For this review, take the finished solid that the model builds, in its own axes (mm). Face numbers are marked on the shaded views. A direction names the side the tool comes from. Give positions to 0.01 mm unless a question says otherwise; leave off trailing zeros. Write each loop counter-clockwise with the first axis right and the second up, starting at its lowest first coordinate (ties: lowest second). Pieces come first, ordered by that corner, then holes.
1) We need section A-A on x = 0. Give the boundary of the cut face in (y, z), and give its area (3 significant figures).
2) Machinability: for the marked faces 1 and 2, which of the approach directions +Z, -Z, +X, -X, +Y, -Y give a long, thin tool a straight path to every point of the face, cutting with its end or side? Answer none if there is none.
3) We need section B-B on z = 0. Give the boundary of the cut face in (x, y).
4) We need section C-C on y = 19. Give the boundary of the cut face in (x, z).
5) Wall thickness on line 1 along Y through (x, z) = (-3, -13); line 2 along Y through (x, z) = (0.75, -8); line 3 along Y through (x, z) = (10.5, -2): over which ranges is each line inside the solid? List them lowest first.
6) For P1, Ø3, axis at x = 6, y = 47, coming from the -Z side; P2, Ø1, axis at x = 5, y = 29.5, coming from the +Z side; P3, Ø8, axis at x = -3.5, z = -11, coming from the +Y side, all flat-tipped, find the tip position at first contact; note any pin that passes through.
7) We need section D-D on y = 50. Give the boundary of the cut face in (x, z), and give its area (3 significant figures).
from build123d import *


with BuildPart() as part:
    # Çizim1 → Döndür1 (revolve)
    with BuildSketch(Plane.XY, mode=Mode.PRIVATE) as d_nd_r1_sk:
        with BuildLine():
            Line((0, 0), (-15, 0))
            Line((-15, 0), (-15, 3))
            Line((-15, 3), (-13, 5))
            ThreePointArc((-13, 5), (-13.688325627, 10.216881481), (-10, 13.97))
            Line((-10, 13.97), (-10, 14.97))
            ThreePointArc((-10, 14.97), (-9.414213562, 16.384213562), (-8, 16.97))
            ThreePointArc((-8, 16.97), (-5.015767327, 28.825089026), (-4.997543238, 41.05))
            ThreePointArc((-4.997543238, 41.05), (-6.411660207, 42.399284866), (-6, 44.31))
            ThreePointArc((-6, 44.31), (-8.407551231, 54.22960274), (0, 60.018203932))
            Line((0, 60.018203932), (0, 0))
        make_face()
    revolve(d_nd_r1_sk.sketch.rotate(Axis((0, 102.341178824, 0), (0, -1, 0)), 270), axis=Axis((0, 102.341178824, 0), (0, -1, 0)))


solid = part.part
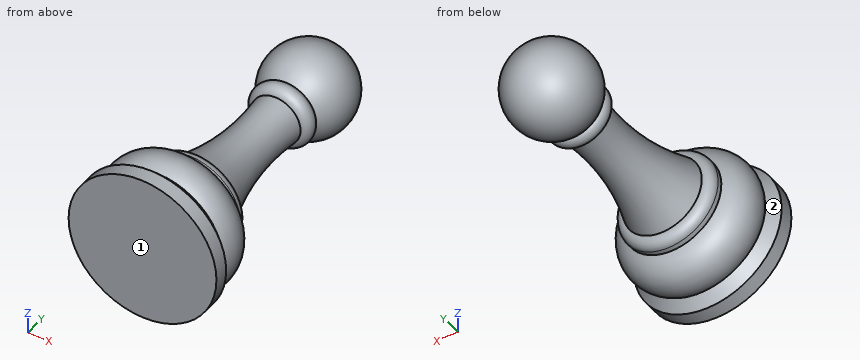
Results list:
1. outline: (0, -15) - (3, -15) - (5, -13) arc R6 ccw to (13.97, -10) - (14.97, -10) arc R2 ccw to (16.97, -8) arc R50 cw to (41.05, -5) arc R2 ccw to (44.31, -6) arc R9 ccw (long way) to (44.31, 6) arc R2 ccw to (41.05, 5) arc R50 cw to (16.97, 8) arc R2 ccw to (14.97, 10) - (13.97, 10) arc R6 ccw to (5, 13) - (3, 15) - (0, 15) - close
1. area: 982 mm2
2. face 1: +Z, -Z, +X, -X, -Y
2. face 2: none
3. outline: (-15, 0) - (15, 0) - (15, 3) - (13, 5) arc R6 ccw to (10, 13.97) - (10, 14.97) arc R2 ccw to (8, 16.97) arc R50 cw to (5, 41.05) arc R2 ccw to (6, 44.31) arc R9 ccw (long way) to (-6, 44.31) arc R2 ccw to (-5, 41.05) arc R50 cw to (-8, 16.97) arc R2 ccw to (-10, 14.97) - (-10, 13.97) arc R6 ccw to (-13, 5) - (-15, 3) - close
4. outline: circle Ø14.53 at (0, 0)
5. line 1: y = 0 to 4.66, 5.58 to 11.04
5. line 2: y = 0 to 16.97, 46.96 to 55.07
5. line 3: y = 0 to 13.68
6. P1: stops at z = -6.95
6. P2: stops at z = 2.04
6. P3: stops at y = 55.93
7. outline: circle Ø17.88 at (0, 0)
7. area: 251 mm2
